```python
from build123d import *

# Parameters (mm, degrees)
F0_W     = 17.272
F0_H     = 10.16
F0_H_2   = 8.670134
F1_DEPTH = 25.4
F2_W     = 32.512
F2_H     = 2.505866
F3_DEPTH = 4.064
F4_R     = 3.81
F5_R     = 1.27
F6_W     = 13.208
F6_H     = 16.51
F7_DEPTH = 21.844
F9_DEPTH = 5.08


with BuildPart() as f1:
    # F0 (on Front) → F1 (new body)
    with BuildSketch(Plane.XZ):
        Polygon((-16.256, 2.505866), (-16.256, 0), (16.256, 0), (16.256, 2.505866), (8.636, 2.505866), (-8.636, 2.505866), align=None)
        with Locations((0, 7.585866)):
            Rectangle(F0_W, F0_H)
        Polygon((-17.78, 12.665866), (-8.636, 12.665866), (8.636, 12.665866), (17.78, 12.665866), (17.78, 22.825866), (8.636, 22.825866), (-8.636, 22.825866), (-17.78, 22.825866), align=None)
        with Locations((0, 27.160933)):
            Rectangle(F0_W, F0_H_2)
    extrude(amount=-F1_DEPTH)

    # F2 (on face) → F3 (join)
    with BuildSketch(Plane(origin=(0, 25.4, 0), x_dir=(-1, 0, 0), z_dir=(0, 1, 0))):
        with Locations((0, 1.252933)):
            Rectangle(F2_W, F2_H)
    extrude(amount=F3_DEPTH)

    # F4
    f4_edges = [f1.edges().sort_by_distance(p)[0] for p in [
        (-8.636, 12.7, 22.825866),
        (-8.636, 12.7, 12.665866),
        (8.636, 12.7, 12.665866),
        (8.636, 12.7, 22.825866),
    ]]
    fillet(f4_edges, radius=F4_R)

    # F5
    f5_edges = [f1.edges().sort_by_distance(p)[0] for p in [
        (-8.636, 12.7, 31.496),
        (8.636, 12.7, 31.496),
        (17.78, 12.7, 22.825866),
        (17.78, 12.7, 12.665866),
        (-17.78, 12.7, 12.665866),
        (-17.78, 12.7, 22.825866),
    ]]
    fillet(f5_edges, radius=F5_R)

    # F6 (on face) → F7 (cut)
    with BuildSketch(Plane.XZ):
        with Locations((0, 17.399)):
            Rectangle(F6_W, F6_H)
    extrude(amount=-F7_DEPTH, mode=Mode.SUBTRACT)

    # F8 (on face) → F9 (cut)
    with BuildSketch(Plane(origin=(0, 0, 0), x_dir=(1, 0, 0), z_dir=(0, 0, -1))):
        with BuildLine():
            ThreePointArc((-14.2875, -25.4254), (-13.640265, -26.987965), (-12.0777, -27.6352))
            Line((-12.0777, -27.6352), (-12.0523, -27.6352))
            ThreePointArc((-12.0523, -27.6352), (-10.489735, -26.987965), (-9.8425, -25.4254))
            Line((-9.8425, -25.4254), (-9.8425, -21.0312))
            ThreePointArc((-9.8425, -21.0312), (-10.489735, -19.468635), (-12.0523, -18.8214))
            Line((-12.0523, -18.8214), (-12.0777, -18.8214))
            ThreePointArc((-12.0777, -18.8214), (-13.640265, -19.468635), (-14.2875, -21.0312))
            Line((-14.2875, -21.0312), (-14.2875, -25.4254))
        make_face()
        with BuildLine():
            Line((12.0777, -18.8214), (12.0523, -18.8214))
            ThreePointArc((12.0523, -18.8214), (10.489735, -19.468635), (9.8425, -21.0312))
            Line((9.8425, -21.0312), (9.8425, -25.4254))
            ThreePointArc((9.8425, -25.4254), (10.489735, -26.987965), (12.0523, -27.6352))
            Line((12.0523, -27.6352), (12.0777, -27.6352))
            ThreePointArc((12.0777, -27.6352), (13.640265, -26.987965), (14.2875, -25.4254))
            Line((14.2875, -25.4254), (14.2875, -21.0312))
            ThreePointArc((14.2875, -21.0312), (13.640265, -19.468635), (12.0777, -18.8214))
        make_face()
    extrude(amount=-F9_DEPTH, mode=Mode.SUBTRACT)


solid = f1.part
```
Model file for the job. Use its own axes, mm. A direction names the side the tool comes from. Give positions to 0.01 mm unless a question says otherwise; leave off trailing zeros. Write each loop counter-clockwise with the first axis right and the second up, starting at its lowest first coordinate (ties: lowest second). Pieces come first, ordered by that corner, then holes. Notation, with made-up numbers: (49, 45.5) -> (71, 45.5) arc R21 ccw to (71, 61.5) -> close; hole circle Ø2 at (35, 85). An arc over 180 degrees is marked (long way). Use CSV: the item, a comma, the result in double quotes. Start each with the question number.
1) Cut at D-D on z = 23.5. List the corners of the cut face in (x, y).
2) Cut at A-A on y = 24. Count the separate pieces of the cut face and the enclosed holes in it, plus the area to 3 significant figures.
3) Cut at C-C on x = -1.5. List the corners of the cut face in (y, z), plus the area to 3 significant figures.
4) Tool access for faces 1 (the flat face through (-14.288, 23, 1)), 2 (the flat face through (0, 25.4, 17)), 3 (the cylindrical face through (-10.5, 27, 1.2)), 4 (the flat face through (14, 13, 12.666)): list every direction of +Z, -Z, +X, -X, +Y, -Y with a clear straight run to the whole face (end or side of a thin tool).
5) Two-plate mould, pull along Z, no slides. Class faces 5 (the flat face through (0, 13, 31.496)), 6 (the flat face through (0, 11, 9.144)), 7 (the flat face through (-8.636, 13, 28)): released by +Z, released by -Z, zero draft, split by the parting line, or undercut.
6) Pin check, flat tips, straight feed: P1, Ø2, axis at x = -14, y = 16, coming from the +Z side; P2, Ø1.8, axis at y = 13, z = 27.5, coming from the +X side; P3, Ø1.3, axis at y = 23.5, z = 1.5, coming from the +X side. Stop position of each tip, or through.
7) Drill centre lines: L1, parallel to Z at x = 1, y = 19.5; L2, parallel to X at y = 8.25, z = 18; L3, parallel to Z at x = 15.5, y = 8.25. Where is each one in solid material? Low to high.
Final values:
1,outline,"(-10.28, 0) -> (-6.6, 0) -> (-6.6, 21.84) -> (6.6, 21.84) -> (6.6, 0) -> (10.28, 0) -> (10.28, 25.4) -> (-10.28, 25.4) -> close"
2,separate pieces,"3"
2,enclosed holes,"0"
2,area,"756 mm2"
3,outline,"(0, 0) -> (29.46, 0) -> (29.46, 2.51) -> (25.4, 2.51) -> (25.4, 31.5) -> (0, 31.5) -> (0, 25.65) -> (21.84, 25.65) -> (21.84, 9.14) -> (0, 9.14) -> close"
3,area,"450 mm2"
4,face 1,"-Z"
4,face 2,"+Z, +X, -X, +Y"
4,face 3,"+Z, -Z"
4,face 4,"+X, +Y, -Y"
5,face 5,"released by +Z"
5,face 6,"undercut"
5,face 7,"zero draft"
6,P1,"stops at z = 22.83"
6,P2,"stops at x = 8.64"
6,P3,"stops at x = 16.26"
7,L1,"z = 0 to 9.14, 25.65 to 31.5"
7,L2,"x = -17.78 to -6.6, 6.6 to 17.78"
7,L3,"z = 0 to 2.51, 12.67 to 22.83"
